Check sheet for the modelled part. Datum: model origin and axes. Units: mm. Face numbers are marked on the shaded views. A direction names the side the tool comes from. Coordinates: 2 decimals unless noted, no trailing zeros. Loops run counter-clockwise (first coordinate to the right, second up) from the corner with the lowest first, then second, coordinate; pieces in that order, holes last.
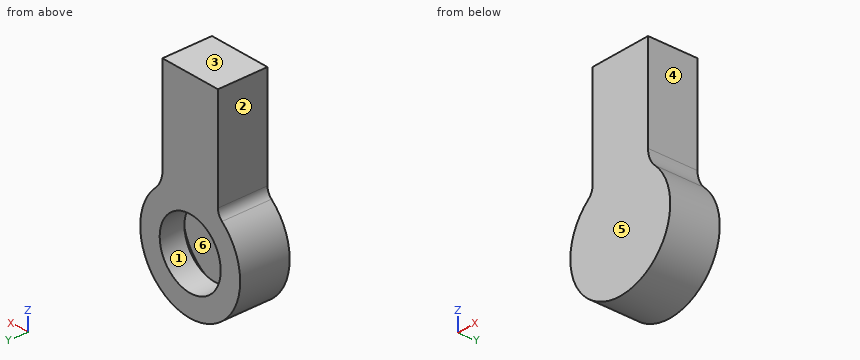
Autodesk Inventor part; units mm, degrees
ref_plane "YZ Plane" through (0, 0, 0) normal (1, 0, 0) x (0, 1, 0)
ref_plane "XZ Plane" through (0, 0, 0) normal (0, 1, 0) x (-1, 0, 0)
ref_plane "XY Plane" through (0, 0, 0) normal (0, 0, 1) x (1, 0, 0)
sketch "Skizze1" plane through (0, 0, 0) normal (0, 1, 0) x (-1, 0, 0)
  line L0 (5, 25) -> (-5, 25)
  line L1 (-5, 25) -> (-5, 9.3808)
  line L2 (5, 8.4853) -> (5, 25)
  arc A0 (-6.2308, 6.4944) -> (5.7273, 6.9425) centre (0, 0) ccw
  arc A1 (5, 8.4853) -> (5.7273, 6.9425) centre (7, 8.4853) ccw
  arc A2 (-6.2308, 6.4944) -> (-5, 9.3808) centre (-9, 9.3808) ccw
  line L3 (0, -16.1968) -> (0, 31.8661)
  point P0 (0, 0)
  point P1 (-5, 7.4833)
  point P2 (5, 7.4833)
  dimension "d2" = 18
  dimension "d3" = 5
  dimension "d4" = 2
  dimension "d5" = 4
  dimension "d8" = 10
  dimension "d9" = 5
  dimension "d10" = 0
  dimension "d11" = 25
extrude "Extrusion1" add sketch "Skizze1" along normal blind 8
sketch "Skizze3" plane through (0, 8, 0) normal (0, 1, 0) x (1, 0, 0)
  circle A0 centre (0, 0) radius 5.5
  dimension "d12" = 11
extrude "Extrusion2" cut sketch "Skizze3" against normal blind 6
sketch "Skizze5" plane through (0, 0, 0) normal (1, 0, 0) x (0, 1, 0)
  line L0 (4, 0) -> (2, 0)
  line L1 (2, 0) -> (2, -8)
  line L2 (4, -6.4) -> (4, 0)
  line L3 (2, 5.5) -> (2, -5.5)
  line L4 (4, -6.4) -> (6.9352, -6.4)
  line L5 (6.9352, -6.4) -> (6.9352, -8)
  line L6 (6.9352, -8) -> (2, -8)
  line L7 (-1.387, 0) -> (8.3222, 0)
  point P0 (0, 0)
  point P1 (3, 0)
  point P2 (5.4676, -6.4)
  dimension "d21" = 0
  dimension "d22" = 2
  dimension "d26" = 8
  dimension "d27" = 6.4
revolve "Umdrehung1" cut sketch "Skizze5" angle 360 about axis through (0, 4, 0) along (0, -1, 0)
properties part number "alternativeJoint"
(1) Gauge pin test, flat ends, axial feed: P1, Ø2, axis at y = 2, z = 18, coming from the +X side; P2, Ø1, axis at y = 7, z = 15.5, coming from the -X side; P3, Ø3, axis at y = 7, z = -3, coming from the +X side. Record the tip position at first contact, or that the pin passes through.
(2) Section check D-D, the plane z = 0. Enter the section's corners in (x, y).
(3) Set-up check for the marked faces 4, 5 and 6: record each of +Z, -Z, +X, -X, +Y, -Y from which the full face is reachable in a straight line by a thin tool's end or side.
(4) Draft check along X on the marked faces 1, 2 and 3. Enter one of: pulls with the +X half, pulls with the -X half, needs draft (parallel to the pull), parting line crosses it, or undercut.
(5) Section check A-A, the plane y = 6.25. Enter the section's corners in (x, z).
(6) Section check B-B, the plane y = 2.5. Enter the section's corners in (x, z).
(7) Scan lines: line 1 along X through (y, z) = (5.15, 0); line 2 along X through (y, z) = (3.45, 0); line 3 along Y through (x, z) = (5.5, 2). Record each from-to range of solid material in increasing order.
(8) Section check C-C, the plane x = 0. Enter the section's corners in (y, z).
Determined:
1. P1: stops at x = 5
1. P2: stops at x = -5
1. P3: stops at x = 8.87
2. outline: (-9, 0) - (9, 0) - (9, 8) - (5.5, 8) - (5.5, 4) - (6.4, 4) - (6.4, 6.94) - (8, 6.94) - (8, 2) - (-8, 2) - (-8, 6.94) - (-6.4, 6.94) - (-6.4, 4) - (-5.5, 4) - (-5.5, 8) - (-9, 8) - close
3. face 4: +Z, +X, +Y, -Y
3. face 5: +Z, -Z, +X, -X, -Y
3. face 6: none
4. face 1: undercut
4. face 2: pulls with the -X half
4. face 3: needs draft
5. outline: circle Ø12.8 at (0, 0); (-5.73, 6.94) arc R9 ccw (long way) to (6.23, 6.49) arc R4 cw to (5, 9.38) - (5, 25) - (-5, 25) - (-5, 8.49) arc R2 cw to start; hole circle Ø16 at (0, 0); hole circle Ø11 at (0, 0)
6. outline: (-5.73, 6.94) arc R9 ccw (long way) to (6.23, 6.49) arc R4 cw to (5, 9.38) - (5, 25) - (-5, 25) - (-5, 8.49) arc R2 cw to start; hole circle Ø16 at (0, 0)
7. line 1: x = -9 to -8, -6.4 to -5.5, 5.5 to 6.4, 8 to 9
7. line 2: x = -9 to -8, 8 to 9
7. line 3: y = 0 to 2, 4 to 8
8. outline: (0, -9) - (8, -9) - (8, -5.5) - (4, -5.5) - (4, -6.4) - (6.94, -6.4) - (6.94, -8) - (2, -8) - (2, 8) - (6.94, 8) - (6.94, 6.4) - (4, 6.4) - (4, 5.5) - (8, 5.5) - (8, 25) - (0, 25) - close
